Read the model definition and answer for the solid it produces. Units are mm, in the model's axes. Face numbers are marked on the shaded views. Coordinates: 2 decimals unless noted, no trailing zeros. Order: outer loops, then holes, each group sorted by start corner. A loop starts at its lowest first (then second) coordinate and runs counter-clockwise, first axis right, second up. Notation, with made-up numbers: M 22,-20 L 28,-20 A28 ccw 28,12 Z; hole C 68,-18 d9. An arc over 180 degrees is marked long. Use a Markdown table: item, result. Add a question column.
1) Find section B-B on y = 21. Write down the section's boundary in (x, z), plus the area to 3 significant figures.
2) The mould has two halves that part along X. Classify the marked faces 1, 2, 3 and 4: released by +X, released by -X, zero draft, split by the parting line, or undercut.
3) Find section D-D on y = 7.5. Write down the section's boundary in (x, z), plus the area to 3 significant figures.
4) This flat-tipped pin is pushed along its axis until it touches: pin 1 Ø4 at (x, y) = (49.5, 28) entering from +Z. Where does it stop, or does it pass through?
5) Find the intervals of material crossed by probe 1 along X at (y, z) = (2, -42); probe 2 along X at (y, z) = (16, -38); probe 3 along Y at (x, z) = (39, -43.5), in increasing order. Write a range as [from, to].
6) Find section C-C on x = 12.5. Write down the section's boundary in (y, z).
7) Find section A-A on z = -32. Write down the section's boundary in (x, y).
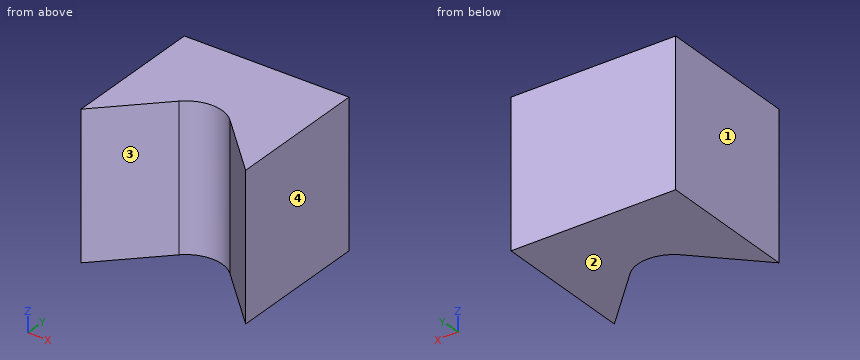
Solid Edge part; units mm, degrees
sketch "Sketch1" plane through (0, 0, 0) normal (0, 0, 1) x (1, 0, 0)
  line L0 (0, 0) -> (57.7, 0)
  line L1 (57.7, 0) -> (57.7, 50)
  line L2 (57.7, 50) -> (0, 50)
  line L3 (0, 50) -> (0, 0)
extrude "Protrusion1" add sketch "Sketch1" against normal blind 50.8
sketch "Sketch2" plane through (28.85, 25, 0) normal (0, 0, 1) x (0, 1, 0)
  line L0 (-25, 28.85) -> (-5.1221, 8.9826)
  arc A0 (-5.1221, 8.9826) -> (-5.1221, -8.9826) centre (-14.1, 0) cw
  line L1 (-25, -28.85) -> (-5.1221, -8.9826)
  line L2 (-25, 28.85) -> (-25, -28.85)
extrude "Recorte_Extrudado_1" cut sketch "Sketch2" against normal blind 50.8
Check result:
| question | item | result |
|---|---|---|
| 1 | outline | M 0,-50.8 L 21.15,-50.8 L 21.15,0 L 0,0 Z; M 36.55,-50.8 L 57.7,-50.8 L 57.7,0 L 36.55,0 Z |
| 1 | area | 2,150 mm2 |
| 2 | face 1 | released by -X |
| 2 | face 2 | zero draft |
| 2 | face 3 | undercut |
| 2 | face 4 | released by +X |
| 3 | outline | M 0,-50.8 L 7.5,-50.8 L 7.5,0 L 0,0 Z; M 50.2,-50.8 L 57.7,-50.8 L 57.7,0 L 50.2,0 Z |
| 3 | area | 762 mm2 |
| 4 | pin 1 | stops at z = 0 |
| 5 | probe 1 | x = [0, 2], [55.7, 57.7] |
| 5 | probe 2 | x = [0, 15.99], [41.71, 57.7] |
| 5 | probe 3 | y = [18.71, 50] |
| 6 | outline | M 12.51,-50.8 L 50,-50.8 L 50,0 L 12.51,0 Z |
| 7 | outline | M 0,0 L 19.87,19.88 A12.7 cw 37.83,19.88 L 57.7,0 L 57.7,50 L 0,50 Z |
